```python
from build123d import *

# Parameters (mm, degrees)
SKETCH_W                     = 11.7
SKETCH_H                     = 11.5
PAD_DEPTH                    = 3.6
PAD001_DEPTH                 = 0.5
PAD001_LINEARPATTERN_2_DEPTH = 0.5
SKETCH002_W                  = 4
SKETCH002_H                  = 0.25
POCKET_DEPTH                 = 11.501
SKETCH003_W                  = 4
SKETCH003_H                  = 0.25
POCKET001_DEPTH              = 11.7
SKETCH005_W                  = 0.5
SKETCH005_H                  = 0.25
POCKET002_DEPTH              = 49.671669
SKETCH006_W                  = 0.5
SKETCH006_H                  = 0.25
POCKET003_DEPTH              = 51.421669
FILLET_R                     = 0.5
SKETCH007_R                  = 3.25
POCKET004_DEPTH              = 1
SKETCH008_W                  = 10.7
SKETCH008_H                  = 10.5
POCKET005_DEPTH              = 0.5
FILLET001_R                  = 1
SKETCH009_R                  = 3.25
PAD002_DEPTH                 = 0.5


with BuildPart() as part:
    # Sketch → Pad (new body)
    with BuildSketch(Plane.XY):
        Rectangle(SKETCH_W, SKETCH_H)
    extrude(amount=PAD_DEPTH)

    # Sketch001 (on DatumPlane) → Pad001 (join, symmetric)
    with BuildSketch(Plane.XZ.offset(2.5)):
        Polygon((-7.4, 0), (-6.8, 0), (-5.85, 0.95), (-5.85, 1.35), (-6.8, 0.4), (-7.4, 0.4), align=None)
    pad001 = extrude(amount=PAD001_DEPTH, both=True)

    # Sketch001 LinearPattern 2 → Pad001 LinearPattern 2 (add, symmetric)
    with BuildSketch(Plane.XZ.offset(-2.5)):
        Polygon((-7.4, 0), (-6.8, 0), (-5.85, 0.95), (-5.85, 1.35), (-6.8, 0.4), (-7.4, 0.4), align=None)
    pad001_linearpattern_2 = extrude(amount=PAD001_LINEARPATTERN_2_DEPTH, both=True)

    # Mirrored: Pad001, Pad001 LinearPattern 2 across Sketch001 V_Axis
    add(pad001.mirror(Plane(origin=(0, -2.5, 0), x_dir=(0, -1, 0), z_dir=(1, 0, 0))))
    add(pad001_linearpattern_2.mirror(Plane(origin=(0, -2.5, 0), x_dir=(0, -1, 0), z_dir=(1, 0, 0))))

    # Sketch002 (on Face6 of MultiTransform) → Pocket (cut, through all)
    with BuildSketch(Plane.XZ.offset(5.75)):
        with Locations((0, 0.125)):
            Rectangle(SKETCH002_W, SKETCH002_H)
    extrude(amount=-POCKET_DEPTH, mode=Mode.SUBTRACT)

    # Sketch003 (on Face7 of Pocket) → Pocket001 (cut)
    with BuildSketch(Plane.YZ.offset(5.85)):
        with Locations((0, 0.125)):
            Rectangle(SKETCH003_W, SKETCH003_H)
    extrude(amount=-POCKET001_DEPTH, mode=Mode.SUBTRACT)

    # Sketch005 (on Face11 of Pocket001) → Pocket002 (cut, through all)
    with BuildSketch(Plane.XZ.offset(5.75)):
        with Locations((5.6, 0.125)):
            Rectangle(SKETCH005_W, SKETCH005_H)
    pocket002 = extrude(amount=-POCKET002_DEPTH, mode=Mode.SUBTRACT)

    # Mirrored001: Pocket002 across Sketch005 V_Axis
    add(pocket002.mirror(Plane(origin=(0, -5.75, 0), x_dir=(0, -1, 0), z_dir=(1, 0, 0))), mode=Mode.SUBTRACT)

    # Sketch006 (on Face11 of Mirrored001) → Pocket003 (cut, through all)
    with BuildSketch(Plane.YZ.offset(5.85)):
        with Locations((-5.5, 0.125)):
            Rectangle(SKETCH006_W, SKETCH006_H)
    pocket003 = extrude(amount=-POCKET003_DEPTH, mode=Mode.SUBTRACT)

    # Mirrored002: Pocket003 across Sketch006 V_Axis
    add(pocket003.mirror(Plane(origin=(5.85, 0, 0), x_dir=(1, 0, 0), z_dir=(0, 1, 0))), mode=Mode.SUBTRACT)

    # Fillet
    fillet_edges = [part.edges().sort_by_distance(p)[0] for p in [
        (5.85, -5.75, 1.925),
        (5.85, 5.75, 1.925),
        (-5.85, -5.75, 1.925),
        (-5.85, 5.75, 1.925),
    ]]
    fillet(fillet_edges, radius=FILLET_R)

    # Sketch007 (on Face5 of Fillet) → Pocket004 (cut)
    with BuildSketch(Plane.XY.offset(3.6)):
        Circle(SKETCH007_R)
    extrude(amount=-POCKET004_DEPTH, mode=Mode.SUBTRACT)

    # Sketch008 (on Face5 of Pocket004) → Pocket005 (cut)
    with BuildSketch(Plane.XY.offset(3.6)):
        Rectangle(SKETCH008_W, SKETCH008_H)
    extrude(amount=-POCKET005_DEPTH, mode=Mode.SUBTRACT)

    # Fillet001
    fillet001_edges = [part.edges().sort_by_distance(p)[0] for p in [
        (-5.35, 5.25, 3.35),
        (5.35, 5.25, 3.35),
        (5.35, -5.25, 3.35),
        (-5.35, -5.25, 3.35),
    ]]
    fillet(fillet001_edges, radius=FILLET001_R)

    # Sketch009 (on Face18 of Fillet001) → Pad002 (join)
    with BuildSketch(Plane.XY.offset(3.1)):
        with BuildLine():
            Line((-3.75, 5.15), (3.75, 5.15))
            ThreePointArc((5.25, 3.65), (4.81066, 4.71066), (3.75, 5.15))
            Line((5.25, 3.65), (5.25, -3.65))
            ThreePointArc((3.75, -5.15), (4.81066, -4.71066), (5.25, -3.65))
            Line((3.75, -5.15), (-3.75, -5.15))
            ThreePointArc((-5.25, -3.65), (-4.81066, -4.71066), (-3.75, -5.15))
            Line((-5.25, -3.65), (-5.25, 3.65))
            ThreePointArc((-3.75, 5.15), (-4.81066, 4.71066), (-5.25, 3.65))
        make_face()
        Circle(SKETCH009_R, mode=Mode.SUBTRACT)
    extrude(amount=PAD002_DEPTH)


solid = part.part
```
The listing builds one solid part. Answer for the finished solid, in the listing's coordinates (mm). A direction names the side the tool comes from. Round coordinates to 2 decimals unless told otherwise and drop trailing zeros. Write each loop counter-clockwise with the first axis right and the second up, starting at its lowest first coordinate (ties: lowest second). Pieces come first, ordered by that corner, then holes. Notation, with made-up numbers: (16, 64) -> (53, 64) arc R19 ccw to (53, 96) -> close; hole circle Ø11 at (-39, 33). An arc over 180 degrees is marked (long way). Use CSV: the item, a comma, the result in double quotes. Start each with the question number.
(1) Consider L1, parallel to Z at x = -1.5, y = -5; L2, parallel to Y at x = 0, z = 2.75; L3, parallel to X at y = 4, z = 2.7. Determine where each line is inside the solid, lowest interval first. Write a range as from..to.
(2) Each of these flat-tipped pins is pushed along its axis until it touches: pin 1 (0.7 mm diameter, centred on x = -7, y = 2.5, fed in from +Z); pin 2 (0.7 mm diameter, centred on x = -7, z = 1, fed in from +Y). Where does it stop, or does it pass through?
(3) Section A-A on z = 2.9 is taken. Give the vertices of the cut face in (x, y).
(4) Section C-C on x = 0 is taken. Give the vertices of the cut face in (y, z), then the cut area to 3 significant figures.
(5) The mould has two halves that part along Y. Classify faces 1 (the face through (0, -5.75, 2)), 2 (the face through (4, 4, 0)), 3 (the face through (-5.049, 4.965, 3.347)): released by +Y, released by -Y, zero draft, split by the parting line, or undercut.
(6) Which of the six approach directions +Z, -Z, +X, -X, +Y, -Y give full straight-line access (tool end or side, diameter ignored) to faces 4 (the face through (-4, 4, 0)), 5 (the face through (5.049, -4.965, 3.347)), 6 (the face through (6.3, 2.5, 0.5))?
(7) Section D-D on y = -4 is taken. Give the vertices of the cut face in (x, z), then the cut area to 3 significant figures.
(8) Section B-B on y = -1.25 is taken. Give the vertices of the cut face in (x, z), then the cut area to 3 significant figures.
A:
1,L1,"z = 0.25..3.6"
1,L2,"y = -5.75..-3.25, 3.25..5.75"
1,L3,"x = -5.85..5.85"
2,pin 1,"stops at z = 0.55"
2,pin 2,"passes through"
3,outline,"(-5.85, -5.25) arc R0.5 ccw to (-5.35, -5.75) -> (5.35, -5.75) arc R0.5 ccw to (5.85, -5.25) -> (5.85, 5.25) arc R0.5 ccw to (5.35, 5.75) -> (-5.35, 5.75) arc R0.5 ccw to (-5.85, 5.25) -> close; hole circle Ø6.5 at (0, 0)"
4,outline,"(-5.75, 0.25) -> (5.75, 0.25) -> (5.75, 3.6) -> (5.25, 3.6) -> (5.25, 3.1) -> (5.15, 3.1) -> (5.15, 3.6) -> (3.25, 3.6) -> (3.25, 2.6) -> (-3.25, 2.6) -> (-3.25, 3.6) -> (-5.15, 3.6) -> (-5.15, 3.1) -> (-5.25, 3.1) -> (-5.25, 3.6) -> (-5.75, 3.6) -> close"
4,area,"31.9 mm²"
5,face 1,"released by -Y"
5,face 2,"zero draft"
5,face 3,"undercut"
6,face 4,"-Z, +X, -X, +Y, -Y"
6,face 5,"+Z"
6,face 6,"-Z, +Y, -Y"
7,outline,"(-5.85, 0.25) -> (-5.35, 0.25) -> (-5.35, 0) -> (-2, 0) -> (-2, 0.25) -> (2, 0.25) -> (2, 0) -> (5.35, 0) -> (5.35, 0.25) -> (5.85, 0.25) -> (5.85, 3.6) -> (5.35, 3.6) -> (5.35, 3.1) -> (5.21, 3.1) -> (5.21, 3.6) -> (-5.21, 3.6) -> (-5.21, 3.1) -> (-5.35, 3.1) -> (-5.35, 3.6) -> (-5.85, 3.6) -> close"
7,area,"40.7 mm²"
8,outline,"(-5.85, 0.25) -> (5.85, 0.25) -> (5.85, 3.6) -> (5.35, 3.6) -> (5.35, 3.1) -> (5.25, 3.1) -> (5.25, 3.6) -> (3, 3.6) -> (3, 2.6) -> (-3, 2.6) -> (-3, 3.6) -> (-5.25, 3.6) -> (-5.25, 3.1) -> (-5.35, 3.1) -> (-5.35, 3.6) -> (-5.85, 3.6) -> close"
8,area,"33.1 mm²"
